Autodesk Inventor part; units mm, degrees
ref_plane "YZ Plane" through (0, 0, 0) normal (1, 0, 0) x (0, 1, 0)
ref_plane "XZ Plane" through (0, 0, 0) normal (0, 1, 0) x (-1, 0, 0)
ref_plane "XY Plane" through (0, 0, 0) normal (0, 0, 1) x (1, 0, 0)
sketch "Sketch1" plane through (0, 0, 0) normal (0, 1, 0) x (-1, 0, 0)
  line L0 (-24.4733, 28.5935) -> (-24.4733, -206.3565)
  line L1 (-24.4733, -206.3565) -> (118.5711, -106.1957)
  line L2 (-24.4733, -206.3565) -> (150.1517, -206.3565) construction
  line L3 (118.5711, -106.1957) -> (118.5711, -42.6957)
  line L4 (118.5711, -42.6957) -> (77.4122, 28.5935)
  line L5 (-24.4733, 28.5935) -> (77.4122, 28.5935)
  point P0 (0, 0)
  dimension "d0" = 234.95
  dimension "d1" = 174.625
  dimension "d2" = 35
  dimension "d3" = 63.5
  dimension "d4" = 150
extrude "Extrusion1" add sketch "Sketch1" along normal blind 3.175
sketch "Sketch2" plane through (0, 0, 0) normal (0, -1, 0) x (1, 0, 0)
  line L0 (24.4733, 28.5935) -> (24.4733, -206.3565)
  line L1 (24.4733, 28.5935) -> (24.4733, -206.3565)
  line L2 (21.2983, -88.8815) -> (21.2983, -69.8315)
  line L3 (21.2983, -88.8815) -> (21.2983, -107.9315)
  line L4 (21.2983, -107.9315) -> (24.4733, -107.9315)
  line L5 (21.2983, -69.8315) -> (24.4733, -69.8315)
  point P0 (0, 0)
  dimension "d8" = 19.05
  dimension "d9" = 19.05
extrude "Extrusion2" add sketch "Sketch2" along normal blind 79.2734
sketch "Sketch3" plane through (24.4733, 3.175, 28.5935) normal (1, 0, 0) x (0, 0, -1)
  line L0 (98.425, -82.4484) -> (117.475, -82.4484)
  line L1 (117.475, -82.4484) -> (117.475, -63.3984)
  line L2 (117.475, -63.3984) -> (98.425, -63.3984)
  line L3 (98.425, -63.3984) -> (98.425, -82.4484)
  point P0 (28.5935, -3.175)
  dimension "d12" = 19.05
  dimension "d13" = 19.05
hole "Hole1" at (24.4733, -60.2234, -88.8815) direction (-1, 0, 0) diameter 8.3312 end through all
properties part number "Left Chest"
The listing builds one solid part. Answer for the finished solid, in the listing's coordinates (mm). Give positions to 0.01 mm unless a question says otherwise; leave off trailing zeros. Write each loop counter-clockwise with the first axis right and the second up, starting at its lowest first coordinate (ties: lowest second). Pieces come first, ordered by that corner, then holes. Notation, with made-up numbers: (85, -6.5) -> (143, -6.5) arc R26 cw to (143, 27.5) -> close; hole circle Ø2 at (29.5, -29). An arc over 180 degrees is marked (long way). Write item = value, one per line. Start each with the question number.
1) Determine the mould class of faces 1 (the face through (-98.28, 1.57, -7.55)), 2 (the face through (-46.048, 1.565, -156.977)), 3 (the face through (22.864, -56.528, -90.804)), 4 (the face through (21.298, -39, -89)) for opening direction Z: +Z half, -Z half, draft (parallel to the pull), parting line (faces both ways), or undercut.
2) Straight lines are drawn through the part: line 1 along Y through (x, z) = (-34, -152) (3 decimals); line 2 along X through (y, z) = (-8, -105.5). For each, find the intervals that lie inside material, in ascending order.
3) The part is cut by section B-B, the plane y = -71.5. Determine the outline of the cut face in (x, z), and give its area (3 significant figures).
4) The part is cut by section A-A, the plane z = -58.5. Determine the outline of the cut face in (x, y) (3 decimals), and give its area (3 significant figures).
5) Each of these flat-tipped pins is pushed along its axis until it touches: pin 1 (1.5 mm diameter, centred on x = -5.5, z = -104.5, fed in from -Y); pin 2 (1.6 mm diameter, centred on x = 22.5, y = -54.5, fed in from +Z); pin 3 (1.6 mm diameter, centred on x = 23.5, y = -49.5, fed in from -Z). Where does it stop, or does it pass through?
Solutions:
q1.face_1 = +Z half
q1.face_2 = -Z half
q1.face_3 = undercut
q1.face_4 = draft
q2.line_1 = 0 to 3.175
q2.line_2 = 21.3 to 24.47
q3.outline = (21.3, -107.93) -> (24.47, -107.93) -> (24.47, -69.83) -> (21.3, -69.83) -> close
q3.area = 121 mm²
q4.outline = (-118.571, 0) -> (24.473, 0) -> (24.473, 3.175) -> (-118.571, 3.175) -> close
q4.area = 454 mm²
q5.pin_1 = 0
q5.pin_2 = -69.83
q5.pin_3 = -107.93
